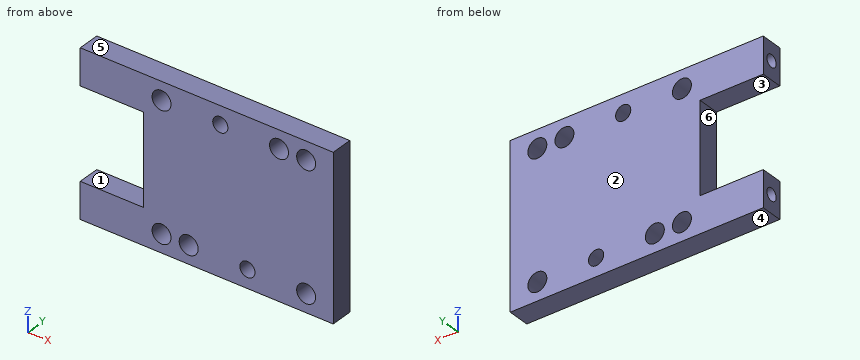
```python
from build123d import *

# Parameters (mm, degrees)
SKETCH1_W                    = 140
SKETCH1_H                    = 90
BOSS_EXTRUDE1_DEPTH          = 12
CUT_EXTRUDE1_REACH           = 86.077
SKETCH2_W                    = 35
SKETCH2_H                    = 50
M10_CLEARANCE_HOLE1_D        = 10.5
F_10_5_10_5_DIAMETER_HOLE1_D = 10.5
M8_TAPPED_HOLE1_D            = 6.8
M8_TAPPED_HOLE1_DEPTH        = 20.207073895
M8_TAPPED_HOLE1_TIP          = 2.042926105
M8_CLEARANCE_HOLE1_D         = 8.4


with BuildPart() as part:
    # Sketch1 → Boss-Extrude1 (new body)
    with BuildSketch(Plane(origin=(0, 0, 0), x_dir=(1, 0, 0), z_dir=(0, 1, 0))):
        Rectangle(SKETCH1_W, SKETCH1_H)
    extrude(amount=-BOSS_EXTRUDE1_DEPTH)

    # Sketch2 → Cut-Extrude1 (cut, up to next)
    with BuildSketch(Plane(origin=(0, 0, 0), x_dir=(1, 0, 0), z_dir=(0, 1, 0)), mode=Mode.PRIVATE) as cut_extrude1_sk1:
        with Locations((-52.5, 0)):
            Rectangle(SKETCH2_W, SKETCH2_H)
    cut_extrude1_tool1 = extrude(cut_extrude1_sk1.sketch, amount=-CUT_EXTRUDE1_REACH, mode=Mode.PRIVATE) & part.part
    add(cut_extrude1_tool1.solids().sort_by_distance((-52.5, 0, 0))[0], mode=Mode.SUBTRACT)

    # M10 Clearance Hole1 (through all)
    with Locations(Plane(origin=(0, 0, 0), x_dir=(1, 0, 0), z_dir=(0, 1, 0))):
        with Locations((-10, 35), (55, 35), (40, -35), (-25, -35)):
            Hole(M10_CLEARANCE_HOLE1_D / 2)

    # Ø10.5 (10.5) Diameter Hole1 (through all)
    with Locations(Plane(origin=(0, 0, 0), x_dir=(1, 0, 0), z_dir=(0, 1, 0))):
        with Locations((-25, 35), (55, -35)):
            Hole(F_10_5_10_5_DIAMETER_HOLE1_D / 2)

    # M8 Tapped Hole1
    with Locations(Plane.ZY.offset(70)):
        with Locations((35, -6), (-35, -6)):
            Hole(M8_TAPPED_HOLE1_D / 2, depth=M8_TAPPED_HOLE1_DEPTH)
            with Locations((0, 0, -(M8_TAPPED_HOLE1_DEPTH + M8_TAPPED_HOLE1_TIP / 2))):  # 118° drill point
                Cone(0, M8_TAPPED_HOLE1_D / 2, M8_TAPPED_HOLE1_TIP, mode=Mode.SUBTRACT)

    # M8 Clearance Hole1 (through all)
    with Locations(Plane(origin=(0, 0, 0), x_dir=(1, 0, 0), z_dir=(0, 1, 0))):
        with Locations((22.5, 35), (7.5, -35)):
            Hole(M8_CLEARANCE_HOLE1_D / 2)


solid = part.part
```
Part model, mm, in its own coordinate system. Face numbers are marked on the shaded views. A direction names the side the tool comes from. Give positions to 0.01 mm unless a question says otherwise; leave off trailing zeros. Loops run counter-clockwise (first coordinate to the right, second up) from the corner with the lowest first, then second, coordinate; pieces in that order, holes last. Notation, with made-up numbers: M 12.5,69 L 47.5,69 A29 cw 47.5,97 Z; hole C -29.75,75.25 d1. An arc over 180 degrees is marked long. Return JSON: item names as keys, results as strings.
1) Saw through at B-B, the plane x = 40. List the corners of the cut face in (y, z).
Calculated:
{"outline": "M -12,-45 L 0,-45 L 0,29.75 L -12,29.75 Z; M -12,40.25 L 0,40.25 L 0,45 L -12,45 Z"}
2) Saw through at D-D, the plane z = 7.5. List the corners of the cut face in (x, y).
Calculated:
{"outline": "M -35,-12 L 70,-12 L 70,0 L -35,0 Z"}
3) Pull direction Z, two halves, no side cores. Call the marked faces 3, 4, 5 and 6: released by +Z, released by -Z, zero draft, split by the parting line, or undercut.
Calculated:
{"face 3": "undercut", "face 4": "released by -Z", "face 5": "released by +Z", "face 6": "undercut"}
4) Saw through at C-C, the plane x = 22.5. List the corners of the cut face in (y, z).
Calculated:
{"outline": "M -12,-45 L 0,-45 L 0,-39.2 L -12,-39.2 Z; M -12,-30.8 L 0,-30.8 L 0,45 L -12,45 Z"}
5) Flat gauge pins, fed straight in: pin 1 Ø8.5 at (x, z) = (55, 35) entering from +Y; pin 2 Ø6 at (y, z) = (-3, -1) entering from -X. Where does each tip first touch, or does it go through?
Calculated:
{"pin 1": "passes through", "pin 2": "stops at x = -35"}
6) Saw through at A-A, the plane x = -25. List the corners of the cut face in (y, z).
Calculated:
{"outline": "M -12,-45 L 0,-45 L 0,-40.25 L -12,-40.25 Z; M -12,-29.75 L 0,-29.75 L 0,29.75 L -12,29.75 Z; M -12,40.25 L 0,40.25 L 0,45 L -12,45 Z"}
7) Drill centre lines: line 1 (Z direction, x = 55, y = -5); line 2 (Z direction, x = -57.5, y = -4.25); line 3 (X direction, y = -5.5, z = -35). Where is each one in solid material? Low to high.
Calculated:
{"line 1": "z = -45 to -40.25, -29.75 to 29.75, 40.25 to 45", "line 2": "z = -45 to -37.92, -32.08 to -25, 25 to 32.08, 37.92 to 45", "line 3": "x = -48.05 to -30.25, -19.75 to -15.25, -4.75 to 18.3, 26.7 to 49.75, 60.25 to 70"}
8) 3-axis set-ups, long thin cutter, end or side, ignore diameter. For the marked faces 1 and 2: which of +Z, -Z, +X, -X, +Y, -Y reach the whole face in a straight line?
Calculated:
{"face 1": "-X, +Y, -Y", "face 2": "+Z, -Z, +X, -X, +Y"}
